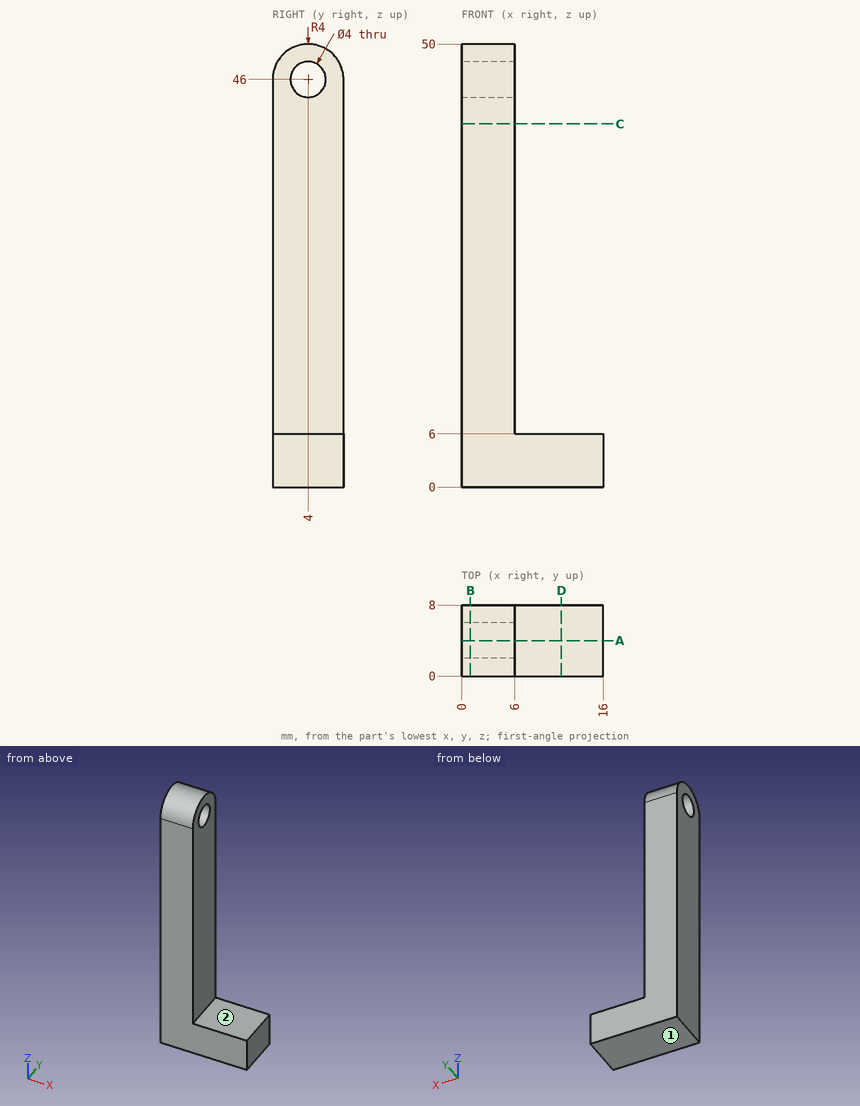
Geometry check sheet. Reference: drawing and pictorial views, mm from the part's lowest x, y, z. A direction names the side the tool comes from. Round coordinates to 2 decimals unless told otherwise and drop trailing zeros. Loops run counter-clockwise (first coordinate to the right, second up) from the corner with the lowest first, then second, coordinate; pieces in that order, holes last. Notation, with made-up numbers: (-40, 42.25) - (-28, 42.25) arc R24 cw to (-28, 52.25) - close; hole circle Ø6 at (-19.5, 70.5). An arc over 180 degrees is marked (long way). Answer in a Markdown table with one row per item. Add a question column.
Q1. Material ranges on line 1 (Y direction, x = 1.35, z = 46); line 2 (X direction, y = 6.5, z = 30), recorded low to high.
Q2. Gauge pin test, flat end, axial feed: pin 1 (4 mm diameter, centred on y = 2, z = 25, fed in from +X). Record the tip position at first contact, or that the pin passes through.
Q3. Section check A-A on y = 4. Enter the section's corners in (x, z), plus the area to 3 significant figures.
Q4. Section check C-C on z = 41. Enter the section's corners in (x, y), plus the area to 3 significant figures.
Q5. Section check D-D on x = 11.25. Enter the section's corners in (y, z), plus the area to 3 significant figures.
Q6. Section check B-B on x = 1. Enter the section's corners in (y, z), plus the area to 3 significant figures.
Q7. Tool access check on the marked faces 1 and 2. Record the directions out of +Z, -Z, +X, -X, +Y, -Y that give a thin tool (end or side, any length) a straight path to the whole face; none if there is none.
Found:
| question | item | result |
|---|---|---|
| 1 | line 1 | y = 0 to 2, 6 to 8 |
| 1 | line 2 | x = 0 to 6 |
| 2 | pin 1 | stops at x = 6 |
| 3 | outline | (0, 0) - (16, 0) - (16, 6) - (6, 6) - (6, 44) - (0, 44) - close; (0, 48) - (6, 48) - (6, 50) - (0, 50) - close |
| 3 | area | 336 mm² |
| 4 | outline | (0, 0) - (6, 0) - (6, 8) - (0, 8) - close |
| 4 | area | 48.0 mm² |
| 5 | outline | (0, 0) - (8, 0) - (8, 6) - (0, 6) - close |
| 5 | area | 48.0 mm² |
| 6 | outline | (0, 0) - (8, 0) - (8, 46) arc R4 ccw to (0, 46) - close; hole circle Ø4 at (4, 46) |
| 6 | area | 381 mm² |
| 7 | face 1 | -Z, +X, -X, +Y, -Y |
| 7 | face 2 | +Z, +X, +Y, -Y |
